from build123d import *

# Parameters (mm, degrees)
SKETCH1_R           = 20
STOCK_DEPTH         = 20
CUT_EXTRUDE1_START  = -10
SKETCH2_OUTSIDE_W   = 54
SKETCH2_OUTSIDE_H   = 54
SKETCH2_OUTSIDE_R   = 15
CUT_EXTRUDE1_DEPTH  = 10
BOSS_EXTRUDE2_START = -20
SKETCH4_R           = 11
BOSS_EXTRUDE2_DEPTH = 10
MAINKEY_START       = -30
SKETCH3_W           = 10
SKETCH3_H           = 22.360679774
MAINKEY_DEPTH       = 20
CENTREBORE_START    = -30
SKETCH5_R           = 7.5
CENTREBORE_DEPTH    = 25
SKETCH6_R           = 3
HOLES_DEPTH         = 23.674794
SKETCH7_R           = 4
CUT_EXTRUDE4_DEPTH  = 1


with BuildPart() as part:
    # Sketch1 → Stock (new body)
    with BuildSketch(Plane(origin=(0, 0, 0), x_dir=(1, 0, 0), z_dir=(0, 1, 0))):
        Circle(SKETCH1_R)
    extrude(amount=-STOCK_DEPTH)

    # Sketch2 outside → Cut-Extrude1 (cut)
    with BuildSketch(Plane(origin=(0, 0, 0), x_dir=(1, 0, 0), z_dir=(0, 1, 0)).offset(CUT_EXTRUDE1_START)):
        Rectangle(SKETCH2_OUTSIDE_W, SKETCH2_OUTSIDE_H)
        Circle(SKETCH2_OUTSIDE_R, mode=Mode.SUBTRACT)
    extrude(amount=-CUT_EXTRUDE1_DEPTH, mode=Mode.SUBTRACT)

    # Sketch4 → Boss-Extrude2 (add)
    with BuildSketch(Plane(origin=(0, 0, 0), x_dir=(1, 0, 0), z_dir=(0, 1, 0)).offset(BOSS_EXTRUDE2_START)):
        Circle(SKETCH4_R)
    extrude(amount=-BOSS_EXTRUDE2_DEPTH)

    # Sketch3 → MainKey (cut)
    with BuildSketch(Plane(origin=(0, 0, 0), x_dir=(1, 0, 0), z_dir=(0, 1, 0)).offset(MAINKEY_START)):
        with Locations((15, 0)):
            Rectangle(SKETCH3_W, SKETCH3_H)
    extrude(amount=MAINKEY_DEPTH, mode=Mode.SUBTRACT)

    # Sketch5 → CentreBore (cut)
    with BuildSketch(Plane(origin=(0, 0, 0), x_dir=(1, 0, 0), z_dir=(0, 1, 0)).offset(CENTREBORE_START)):
        Circle(SKETCH5_R)
    extrude(amount=CENTREBORE_DEPTH, mode=Mode.SUBTRACT)

    # Sketch6 → Holes (cut)
    with BuildSketch(Plane(origin=(10, 0, 0), x_dir=(0, 0, -1), z_dir=(1, 0, 0))):
        with Locations((0, -25)):
            Circle(SKETCH6_R)
    extrude(amount=-HOLES_DEPTH, mode=Mode.SUBTRACT)

    # Sketch7 → Cut-Extrude4 (cut)
    with BuildSketch(Plane(origin=(10, 0, 0), x_dir=(0, 0, -1), z_dir=(1, 0, 0))):
        with Locations((0, -25)):
            Circle(SKETCH7_R)
    extrude(amount=-CUT_EXTRUDE4_DEPTH, mode=Mode.SUBTRACT)


solid = part.part
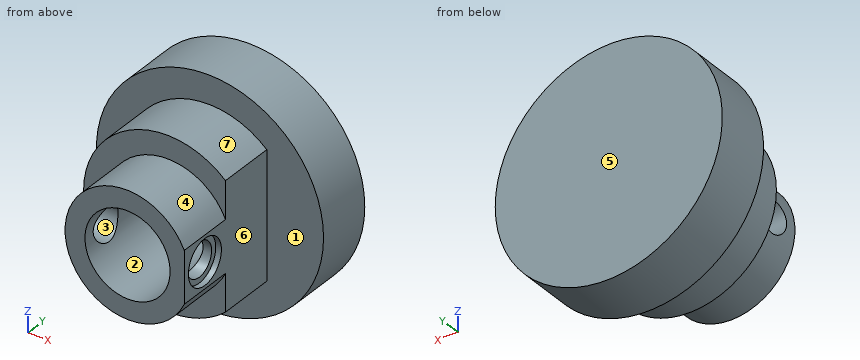
CAD build for the part. Positions are in the model's coordinates, mm. Face numbers are marked on the shaded views. A direction names the side the tool comes from. Round coordinates to 2 decimals unless told otherwise and drop trailing zeros. Order: outer loops, then holes, each group sorted by start corner. A loop starts at its lowest first (then second) coordinate and runs counter-clockwise, first axis right, second up. Notation, with made-up numbers: (-29.75, 79) - (-20.75, 79) arc R21 ccw to (-20.75, 83) - close; hole circle Ø11 at (84, -10). An arc over 180 degrees is marked (long way). Return JSON: item names as keys, results as strings.
(1) Pull direction Z, two halves, no side cores. Call the marked faces 1, 2, 3 and 4: +Z half, -Z half, draft (parallel to the pull), parting line (faces both ways), or undercut.
Answer key:
{"face 1": "draft", "face 2": "undercut", "face 3": "undercut", "face 4": "parting line"}
(2) Cut at C-C (y = -25). Give the cut face in (x, z), then the cut area to 3 significant figures.
Answer key:
{"outline": "(-10.58, -3) arc R11 ccw to (10, -4.58) - (10, -4) - (9, -4) - (9, -3) - (6.87, -3) arc R7.5 cw to (-6.87, -3) - close; (-10.58, 3) - (-6.87, 3) arc R7.5 cw to (6.87, 3) - (9, 3) - (9, 4) - (10, 4) - (10, 4.58) arc R11 ccw to start", "area": "158 mm^2"}
(3) Tool access for the marked faces 5, 6 and 7: list every direction of +Z, -Z, +X, -X, +Y, -Y with a clear straight run to the whole face (end or side of a thin tool).
Answer key:
{"face 5": "+Z, -Z, +X, -X, +Y", "face 6": "+Z, -Z, +X, -Y", "face 7": "-Y"}
(4) Cut at A-A (z = 0). Give the cut face in (x, y), then the cut area to 3 significant figures.
Answer key:
{"outline": "(-20, -10) - (-15, -10) - (-15, -20) - (-11, -20) - (-11, -22) - (-7.5, -22) - (-7.5, -5) - (7.5, -5) - (7.5, -22) - (9, -22) - (9, -21) - (10, -21) - (10, -10) - (20, -10) - (20, 0) - (-20, 0) - close; (-11, -30) - (-7.5, -30) - (-7.5, -28) - (-11, -28) - close; (7.5, -30) - (10, -30) - (10, -29) - (9, -29) - (9, -28) - (7.5, -28) - close", "area": "447 mm^2"}
(5) Pin check, flat tips, straight feed: pin 1 Ø10 at (x, y) = (-3, -25.5) entering from +Z; pin 2 Ø8 at (y, z) = (-25, 0) entering from -X; pin 3 Ø12 at (x, z) = (0, 0) entering from +Y; pin 4 Ø4 at (x, y) = (6, -9.5) entering from +Z. Stop position of each tip, or through.
Answer key:
{"pin 1": "stops at z = 11", "pin 2": "stops at x = -11", "pin 3": "stops at y = 0", "pin 4": "stops at z = 19.6"}
(6) Wall check: probe 1 along Y at (x, z) = (-8, 0); probe 2 along Z at (x, y) = (0, -22); probe 3 along Y at (x, z) = (9.4, 0). Give the ranges that are in metal, low to high. Write a range as from..to.
Answer key:
{"probe 1": "y = -30..-28, -22..0", "probe 2": "z = -11..-7.5, 7.5..11", "probe 3": "y = -30..-29, -21..0"}
(7) Cut at B-B (x = 0). Give the cut face in (y, z).
Answer key:
{"outline": "(-30, -11) - (-20, -11) - (-20, -15) - (-10, -15) - (-10, -20) - (0, -20) - (0, 20) - (-10, 20) - (-10, 15) - (-20, 15) - (-20, 11) - (-30, 11) - (-30, 7.5) - (-5, 7.5) - (-5, -7.5) - (-30, -7.5) - close"}
(8) Cut at D-D (z = -12). Give the cut face in (x, y).
Answer key:
{"outline": "(-16, -10) - (-9, -10) - (-9, -20) - (9, -20) - (9, -10) - (16, -10) - (16, 0) - (-16, 0) - close"}
